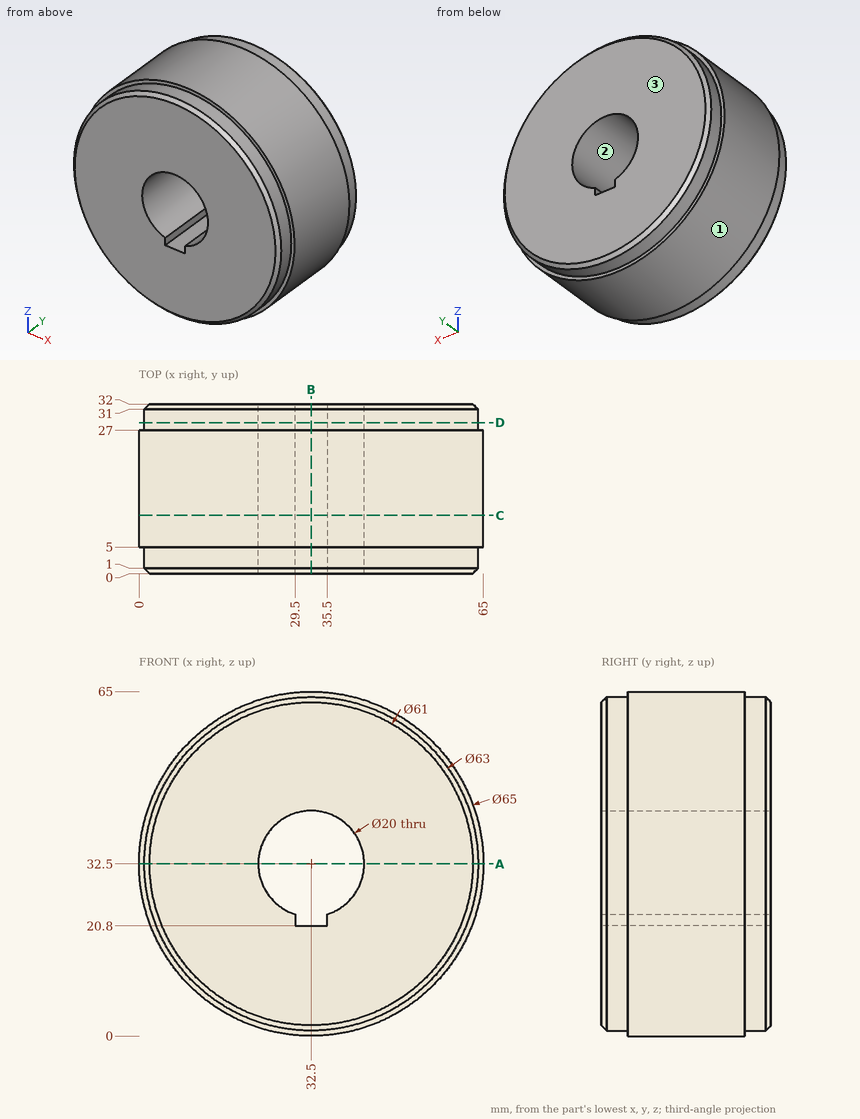
Answer from the drawing. Dimensions are ordinates in mm from the lowest x, y and z of the part. Round coordinates to 2 decimals unless told otherwise and drop trailing zeros. Write each loop counter-clockwise with the first axis right and the second up, starting at its lowest first coordinate (ties: lowest second). Pieces come first, ordered by that corner, then holes. Notation, with made-up numbers: M 62.5,89 L 100.5,89 A25 ccw 100.5,110 Z; hole C 15.25,60.5 d7. An arc over 180 degrees is marked long. Write each question's results on one line, items separated by ' | '. Start each with the question number.
Item 1: Find section C-C on y = 11. Write down the section's boundary in (x, z).
Item 2: Find section D-D on y = 28.5. Write down the section's boundary in (x, z), and give its area (3 significant figures).
Item 3: Straight lines are drawn through the part: probe 1 along X at (y, z) = (17.5, 32.5); probe 2 along Z at (x, y) = (32, 18); probe 3 along Z at (x, y) = (36, 7). For each, find the intervals that lie inside material, in ascending order.
Item 4: Given pin 1 Ø8 at (y, z) = (18, 8.5) entering from +X; pin 2 Ø2.5 at (y, z) = (18.5, 22) entering from +X; pin 3 Ø6 at (x, y) = (45.5, 20.5) entering from -Z, each flat-ended and moving along its own axis, determine where each tip first touches the part or whether it passes through.
Item 5: Find section A-A on z = 32.5. Write down the section's boundary in (x, y).
Item 6: The mould has two halves that part along X. Classify the marked faces 1, 2 and 3: +X half, -X half, draft (parallel to the pull), parting line (faces both ways), or undercut.
Item 7: Find section B-B on x = 32.5. Write down the section's boundary in (y, z), and give its area (3 significant figures).
Answer block:
1) outline: C 32.5,32.5 d65; hole M 29.5,20.8 L 35.5,20.8 L 35.5,22.96 A10 ccw long 29.5,22.96 Z
2) outline: C 32.5,32.5 d63; hole M 29.5,20.8 L 35.5,20.8 L 35.5,22.96 A10 ccw long 29.5,22.96 Z | area: 2,790 mm²
3) probe 1: x = 0 to 22.5, 42.5 to 65 | probe 2: z = 0 to 20.8, 42.49 to 65 | probe 3: z = 0.19 to 23.13, 41.87 to 64.81
4) pin 1: stops at x = 58.12 | pin 2: stops at x = 63.66 | pin 3: stops at z = 1.58
5) outline: M 0,5 L 1,5 L 1,1 L 2,0 L 22.5,0 L 22.5,32 L 2,32 L 1,31 L 1,27 L 0,27 Z; M 42.5,0 L 63,0 L 64,1 L 64,5 L 65,5 L 65,27 L 64,27 L 64,31 L 63,32 L 42.5,32 Z
6) face 1: parting line | face 2: undercut | face 3: draft
7) outline: M 0,2 L 1,1 L 5,1 L 5,0 L 27,0 L 27,1 L 31,1 L 32,2 L 32,20.8 L 0,20.8 Z; M 0,42.5 L 32,42.5 L 32,63 L 31,64 L 27,64 L 27,65 L 5,65 L 5,64 L 1,64 L 0,63 Z | area: 1,360 mm²
